Can you work these out from the model? Positions are in its coordinate system, mm. A direction names the side the tool comes from. Round coordinates to 2 decimals unless told otherwise and drop trailing zeros. Loops run counter-clockwise (first coordinate to the right, second up) from the corner with the lowest first, then second, coordinate; pieces in that order, holes last. Notation, with made-up numbers: (1, 59.5) -> (6, 59.5) arc R33 ccw to (6, 94.5) -> close; hole circle Ø11 at (44.5, 16.25). An arc over 180 degrees is marked (long way). Write item = value, one per line.
from build123d import *

# Parameters (mm, degrees)
SKETCH1_R           = 25
BOSS_EXTRUDE1_DEPTH = 65
CHAMFER1_SIZE       = 6
SKETCH2_R           = 4
BOSS_EXTRUDE2_DEPTH = 16
BOSS_EXTRUDE3_START = 23
SKETCH4_R           = 4
BOSS_EXTRUDE3_DEPTH = 23
CUT_EXTRUDE4_DEPTH  = 20
SKETCH6_R           = 2
CUT_EXTRUDE5_DEPTH  = 20
CUT_EXTRUDE6_START  = -10
SKETCH7_R           = 25
SKETCH7_R_2         = 10
CUT_EXTRUDE6_DEPTH  = 1


with BuildPart() as part:
    # Sketch1 → Boss-Extrude1 (new body)
    with BuildSketch(Plane(origin=(0, 0, 0), x_dir=(1, 0, 0), z_dir=(0, 1, 0))):
        with Locations(Location((0, 0, 0), (0, 0, 270))):
            Circle(SKETCH1_R)
    extrude(amount=BOSS_EXTRUDE1_DEPTH)

    # Chamfer1
    chamfer1_edges = [part.edges().sort_by_distance(p)[0] for p in [
        (0, 0, -25),
        (0, 65, -25),
    ]]
    chamfer(chamfer1_edges, length=CHAMFER1_SIZE)

    # Sketch2 → Boss-Extrude2 (add)
    with BuildSketch(Plane(origin=(0, 65, 0), x_dir=(1, 0, 0), z_dir=(0, 1, 0))):
        with Locations(Location((0, 0, 0), (0, 0, 270))):
            Circle(SKETCH2_R)
    extrude(amount=BOSS_EXTRUDE2_DEPTH)

    # Sketch4 → Boss-Extrude3 (add)
    with BuildSketch(Plane.XZ.offset(BOSS_EXTRUDE3_START)):
        with Locations(Location((0, 0, 0), (0, 0, 90))):
            Circle(SKETCH4_R)
    extrude(amount=-BOSS_EXTRUDE3_DEPTH)

    # Sketch5 → Cut-Extrude4 (cut)
    with BuildSketch(Plane.XZ.offset(23)):
        with BuildLine():
            Line((-1.936491673, 3.5), (1.936491673, 3.5))
            ThreePointArc((1.936491673, 3.5), (0, 4), (-1.936491673, 3.5))
        make_face()
    extrude(amount=-CUT_EXTRUDE4_DEPTH, mode=Mode.SUBTRACT)

    # Sketch6 → Cut-Extrude5 (cut)
    with BuildSketch(Plane(origin=(0, 0, 0), x_dir=(-1, 0, 0), z_dir=(0, -1, 0))):
        with Locations(Location((15, 0, 0), (0, 0, 90))):
            Circle(SKETCH6_R)
        with Locations(Location((0, -15, 0), (0, 0, 90))):
            Circle(SKETCH6_R)
        with Locations(Location((-15, 0, 0), (0, 0, 90))):
            Circle(SKETCH6_R)
        with Locations(Location((0, 15, 0), (0, 0, 90))):
            Circle(SKETCH6_R)
    extrude(amount=-CUT_EXTRUDE5_DEPTH, mode=Mode.SUBTRACT)

    # Sketch7 → Cut-Extrude6 (cut)
    with BuildSketch(Plane.XZ.offset(CUT_EXTRUDE6_START)):
        with Locations(Location((0, 0, 0), (0, 0, 270))):
            Circle(SKETCH7_R)
        with Locations(Location((0, 0, 0), (0, 0, 270))):
            Circle(SKETCH7_R_2, mode=Mode.SUBTRACT)
    extrude(amount=-CUT_EXTRUDE6_DEPTH, mode=Mode.SUBTRACT)


solid = part.part
1. We'd pull the mould along Z, two halves only. Please class faces 1 (the cylindrical face through (-3.905, 72.888, -0.867)), 2 (the flat face through (15, 20, 0)), 3 (the flat face through (4.5, 0, -0.3)): released by +Z, released by -Z, zero draft, split by the parting line, or undercut.
Entries:
face_1 = split by the parting line
face_2 = undercut
face_3 = zero draft
2. For faces 4 (the flat face through (0, -23, 0)), 5 (the flat face through (-11, 11, 0)), 6 (the cylindrical face through (-13, 15, 0)), which set-ups out of +Z, -Z, +X, -X, +Y, -Y let a thin tool reach every point of the face, with its end or its side?
Entries:
face_4 = +Z, -Z, +X, -X, -Y
face_5 = none
face_6 = -Y
3. Suppose I cut it at D-D, the plane y = 56. List the corners of the cut face in (x, z) for me, and give its area (3 significant figures).
Entries:
outline = circle Ø50 at (0, 0)
area = 1,960 mm²
4. Suppose I cut it at B-B, the plane y = -12.5. List the corners of the cut face in (x, z) for me.
Entries:
outline = (-1.94, 3.5) arc R4 ccw (long way) to (1.94, 3.5) -> close
5. Suppose I cut it at A-A, the plane x = 0. Count the separate pieces of the cut face and the enclosed holes in it, and give its area (3 significant figures).
Entries:
separate_pieces = 3
enclosed_holes = 0
area = 3,300 mm²
6. I'm going to push flat-ended pins straight in: pin 1 (6 mm diameter, centred on x = 9.5, z = 15.5, fed in from +Y); pin 2 (10 mm diameter, centred on y = 40.5, z = -14.5, fed in from -X); pin 3 (2.5 mm diameter, centred on x = 0, z = -15, fed in from -Y). Where does each tip first touch, or does it pass through?
Entries:
pin_1 = 65
pin_2 = -23.12
pin_3 = 20
7. I need wall thicknesses on line 1 (X direction, y = 17, z = 0); line 2 (Y direction, x = 10, z = -11); line 3 (X direction, y = 13.5, z = 15). Which ranges of each line are inside material? Lowest first, please. Write a range as [from, to].
Entries:
line_1 = [-25, -17], [-13, 13], [17, 25]
line_2 = [0, 10], [11, 65]
line_3 = [-20, -2], [2, 20]
